Geometry: final body of the model. Coordinates: model frame, mm. A direction names the side the tool comes from. Give positions to 0.01 mm unless a question says otherwise; leave off trailing zeros. Write each loop counter-clockwise with the first axis right and the second up, starting at its lowest first coordinate (ties: lowest second). Pieces come first, ordered by that corner, then holes.
```python
from build123d import *

# Parameters (mm, degrees)
SKETCH_2_W          = 30
SKETCH_2_H          = 30
EXTRUDE_1_DEPTH     = 2
SKETCH_3_W          = 30
SKETCH_3_H          = 20
EXTRUDE_2_DEPTH     = 4
SKETCH_6_R          = 1.525
CUT_EXTRUDE_1_DEPTH = 80
SKETCH_7_W          = 16
SKETCH_7_H          = 12
EXTRUDE_3_DEPTH     = 4
SKETCH_9_R          = 1.525
CUT_EXTRUDE_2_DEPTH = 4
FILLET_2_R          = 2


with BuildPart() as part:
    # 草图2 → 凸台-拉伸1 (new body, symmetric)
    with BuildSketch(Plane.XY):
        Rectangle(SKETCH_2_W, SKETCH_2_H)
    extrude(amount=EXTRUDE_1_DEPTH, both=True)

    # 草图3 → 凸台-拉伸2 (add)
    with BuildSketch(Plane.XY.offset(2)):
        with Locations((0, -25)):
            Rectangle(SKETCH_3_W, SKETCH_3_H)
    extrude(amount=-EXTRUDE_2_DEPTH)

    # 草图6 → 切除-拉伸1 (cut)
    with BuildSketch(Plane.XY.offset(2)):
        with Locations((1, -9.7)):
            Circle(SKETCH_6_R)
        with Locations((-11, 2.3)):
            Circle(SKETCH_6_R)
        with Locations((-10, 12)):
            Circle(SKETCH_6_R)
        with Locations((10, 12)):
            Circle(SKETCH_6_R)
    extrude(amount=-CUT_EXTRUDE_1_DEPTH, mode=Mode.SUBTRACT)

    # 草图7 → 凸台-拉伸3 (add)
    with BuildSketch(Plane.XY.offset(2)):
        with Locations((-23, -29)):
            Rectangle(SKETCH_7_W, SKETCH_7_H)
    extrude(amount=-EXTRUDE_3_DEPTH)

    # 草图9 → 切除-拉伸2 (cut)
    with BuildSketch(Plane(origin=(0, 0, -2), x_dir=(-1, 0, 0), z_dir=(0, 0, -1))):
        with Locations((3, -28)):
            Circle(SKETCH_9_R)
        with Locations((23, -28)):
            Circle(SKETCH_9_R)
    extrude(amount=-CUT_EXTRUDE_2_DEPTH, mode=Mode.SUBTRACT)

    # 圆角2
    fillet_2_edges = [part.edges().sort_by_distance(p)[0] for p in [
        (15, -35, 0),
        (-31, -23, 0),
        (-31, -35, 0),
        (-15, -23, 0),
        (-15, 15, 0),
        (15, 15, 0),
    ]]
    fillet(fillet_2_edges, radius=FILLET_2_R)


solid = part.part
```
Item 1: Section C-C, the plane z = 0.3. Return the cut outline in (x, y) (3 decimals), plus the area to 3 significant figures.
Found:
outline: (-31, -33) arc R2 ccw to (-29, -35) - (13, -35) arc R2 ccw to (15, -33) - (15, 13) arc R2 ccw to (13, 15) - (-13, 15) arc R2 ccw to (-15, 13) - (-15, -21) arc R2 cw to (-17, -23) - (-29, -23) arc R2 ccw to (-31, -25) - close; hole circle Ø3.05 at (-23, -28); hole circle Ø3.05 at (-11, 2.3); hole circle Ø3.05 at (-10, 12); hole circle Ø3.05 at (-3, -28); hole circle Ø3.05 at (1, -9.7); hole circle Ø3.05 at (10, 12)
area: 1,640 mm2
Item 2: Pin query (flat end, axial travel): pin 1 Ø2 at (y, z) = (-20.5, -1) entering from -X; pin 2 Ø1.2 at (x, z) = (-23, -1) entering from +Y; pin 3 Ø2 at (y, z) = (-10, 1) entering from -X. Return the tip coordinate at first contact, or that it passes through.
Found:
pin 1: stops at x = -15.06
pin 2: stops at y = -23
pin 3: stops at x = -15
Item 3: Line query: L1, parallel to Y at x = 1, z = -0.9 (3 decimals); L2, parallel to Y at x = -10, z = 0.4 (3 decimals); L3, parallel to Y at x = 10, z = -0.25 (3 decimals). Output: solid intervals per line, ascending.
Found:
L1: y = -35 to -11.225, -8.175 to 15
L2: y = -35 to 1.149, 3.451 to 10.475, 13.525 to 15
L3: y = -35 to 10.475, 13.525 to 15
Item 4: Section A-A, the plane y = -9.7. Return the cut outline in (x, z) (3 decimals), plus the area to 3 significant figures.
Found:
outline: (-15, -2) - (-0.525, -2) - (-0.525, 2) - (-15, 2) - close; (2.525, -2) - (15, -2) - (15, 2) - (2.525, 2) - close
area: 108 mm2
Item 5: Section B-B, the plane y = 12. Return the cut outline in (x, z) (3 decimals).
Found:
outline: (-15, -2) - (-11.525, -2) - (-11.525, 2) - (-15, 2) - close; (-8.475, -2) - (8.475, -2) - (8.475, 2) - (-8.475, 2) - close; (11.525, -2) - (15, -2) - (15, 2) - (11.525, 2) - close
Item 6: Section D-D, the plane x = 10. Return the cut outline in (y, z) (3 decimals), plus the area to 3 significant figures.
Found:
outline: (-35, -2) - (10.475, -2) - (10.475, 2) - (-35, 2) - close; (13.525, -2) - (15, -2) - (15, 2) - (13.525, 2) - close
area: 188 mm2
Item 7: Reachability of faces 1 (the face through (-23, -23, 0)), 2 (the face through (-8, -35, 0)) from +Z, -Z, +X, -X, +Y, -Y: full face, straight path, thin tool, end or side. Return the list, or none.
Found:
face 1: +Z, -Z, -X, +Y
face 2: +Z, -Z, +X, -X, -Y
Item 8: Pull-direction query (Y, two-part tool) for faces 3 (the face through (-8.6, 11.4, 0)), 4 (the face through (-30.43, -23.6, -0.03)), 5 (the face through (14.4, -34.43, -0.03)); classes: +Y half, -Y half, draft (parallel to the pull), parting line (faces both ways), or undercut.
Found:
face 3: undercut
face 4: +Y half
face 5: -Y half
